```python
from build123d import *

# Parameters (mm, degrees)
SKETCH1_R           = 40
BOSS_EXTRUDE1_DEPTH = 5
CUT_EXTRUDE3_START  = -10
CUT_EXTRUDE3_DEPTH  = 10
FILLET1_R           = 30
FILLET2_R           = 25
SKETCH14_W          = 7
SKETCH14_H          = 5.05
CUT_EXTRUDE4_DEPTH  = 10
SKETCH18_W          = 10
SKETCH18_H          = 7
CUT_EXTRUDE6_DEPTH  = 10
SKETCH20_R          = 8.5
CUT_EXTRUDE8_DEPTH  = 1


with BuildPart() as part:
    # Sketch1 → Boss-Extrude1 (new body)
    with BuildSketch(Plane.XY):
        Circle(SKETCH1_R)
    extrude(amount=BOSS_EXTRUDE1_DEPTH)

    # Sketch10 → Cut-Extrude3 (cut)
    with BuildSketch(Plane.XY.offset(5).offset(CUT_EXTRUDE3_START)):
        with BuildLine():
            Line((-30, 26.457513111), (-30, -26.457513111))
            ThreePointArc((-30, -26.457513111), (-40, 0), (-30, 26.457513111))
        make_face()
        with BuildLine():
            Line((30, 26.457513111), (30, -26.457513111))
            ThreePointArc((30, -26.457513111), (40, 0), (30, 26.457513111))
        make_face()
    extrude(amount=CUT_EXTRUDE3_DEPTH, mode=Mode.SUBTRACT)

    # Fillet1
    fillet1_edges = [part.edges().sort_by_distance(p)[0] for p in [
        (-30, 26.457513111, 2.5),
        (30, 26.457513111, 2.5),
    ]]
    fillet(fillet1_edges, radius=FILLET1_R - 0.0001)  # a hair under: the kernel refuses the full size

    # Fillet2
    fillet2_edges = [part.edges().sort_by_distance(p)[0] for p in [
        (-30, -26.457513111, 2.5),
        (30, -26.457513111, 2.5),
    ]]
    fillet(fillet2_edges, radius=FILLET2_R)

    # Sketch14 → Cut-Extrude4 (cut)
    with BuildSketch(Plane.XY.offset(5)):
        with Locations((0, 1.975)):
            Rectangle(SKETCH14_W, SKETCH14_H)
        with Locations((0, -18.075)):
            Rectangle(SKETCH14_W, SKETCH14_H)
    extrude(amount=-CUT_EXTRUDE4_DEPTH, mode=Mode.SUBTRACT)

    # Sketch18 → Cut-Extrude6 (cut)
    with BuildSketch(Plane(origin=(0, 0, 0), x_dir=(-1, 0, 0), z_dir=(0, 0, -1))):
        with Locations((-18, -7)):
            Rectangle(SKETCH18_W, SKETCH18_H)
    extrude(amount=-CUT_EXTRUDE6_DEPTH, mode=Mode.SUBTRACT)

    # Sketch20 → Cut-Extrude8 (cut)
    with BuildSketch(Plane(origin=(0, 0, 0), x_dir=(-1, 0, 0), z_dir=(0, 0, -1))):
        with Locations((-17.5, 20)):
            Circle(SKETCH20_R)
        with Locations((17.5, 20)):
            Circle(SKETCH20_R)
        with Locations((17.5, -20)):
            Circle(SKETCH20_R)
        with Locations((-17.5, -20)):
            Circle(SKETCH20_R)
    extrude(amount=-CUT_EXTRUDE8_DEPTH, mode=Mode.SUBTRACT)


solid = part.part
```
Could you check a few things on this model? Use its own coordinates, in mm. A direction names the side the tool comes from. Coordinates: 2 decimals unless noted, no trailing zeros. Order: outer loops, then holes, each group sorted by start corner. A loop starts at its lowest first (then second) coordinate and runs counter-clockwise, first axis right, second up. Notation, with made-up numbers: M -12,47 L -8,47 A6 cw -8,54 Z; hole C -1,-27 d1. An arc over 180 degrees is marked long. Use one line per item in the form item = value. Start each with the question number.
1. Suppose I cut it at D-D on x = -17.5. Write out the boundary of the cut face in (y, z), then the cut area to 3 significant figures.
2. For pin 1 (3 mm diameter, centred on y = 17.5, z = 3.5, fed in from +X); pin 2 (5 mm diameter, centred on x = -19, y = 24, fed in from -Z); pin 3 (2.5 mm diameter, centred on y = -17.5, z = 2, fed in from +X), each with a flat end and sliding along its axis, tell me the tip position at first contact or that it passes through.
3. Suppose I cut it at C-C on y = 20. Write out the boundary of the cut face in (x, z).
4. Please list where these lines run through material, in increasing order: line 1 (Y direction, x = -17.5, z = 0.8); line 2 (Y direction, x = 2, z = 3.1); line 3 (X direction, y = 1, z = 2.25).
5. Suppose I cut it at B-B on x = 17.5. Write out the boundary of the cut face in (y, z), then the cut area to 3 significant figures.
6. On a 3-axis mill with a long thin cutter (end or side, diameter ignored), from which of +Z, -Z, +X, -X, +Y, -Y can I reach the whole of each face in a straight line? I mean faces 4 (the cylindrical face through (-10.755, 14.828, 0.493)), 5 (the flat face through (18, -3.5, 2)), 6 (the cylindrical face through (20.979, 31.445, 2.535)). Say none if no direction works.
7. Suppose I cut it at A-A on z = 2.3. Count the separate pieces of the cut face and the enclosed holes in it, then the cut area to 3 significant figures.
8. We'd pull the mould along Y, two halves only. Please class faces 1 (the flat face through (6, 1, 0)), 2 (the flat face through (0, 4.5, 3)), 3 (the cylindrical face through (-20.979, 31.445, 2.535)): +Y half, -Y half, draft (parallel to the pull), parting line (faces both ways), or undercut.
Geometry says:
q1.outline = M -35.79,0 L -28.5,0 L -28.5,1 L -11.5,1 L -11.5,0 L 11.5,0 L 11.5,1 L 28.5,1 L 28.5,0 L 34.37,0 L 34.37,5 L -35.79,5 Z
q1.area = 317 mm^2
q2.pin_1 = 29.39
q2.pin_2 = 1
q2.pin_3 = 29.91
q3.outline = M -28.28,0 L -26,0 L -26,1 L -9,1 L -9,0 L 9,0 L 9,1 L 26,1 L 26,0 L 28.28,0 L 28.28,5 L -28.28,5 Z
q4.line_1 = -35.79 to -28.5, -11.5 to 11.5, 28.5 to 34.37
q4.line_2 = -39.95 to -20.6, -15.55 to -0.55, 4.5 to 39.93
q4.line_3 = -30 to -3.5, 3.5 to 30
q5.outline = M -35.79,0 L -28.5,0 L -28.5,1 L -11.5,1 L -11.5,0 L -10.5,0 L -10.5,5 L -35.79,5 Z; M -3.5,0 L 11.5,0 L 11.5,1 L 28.5,1 L 28.5,0 L 34.37,0 L 34.37,5 L -3.5,5 Z
q5.area = 282 mm^2
q6.face_4 = -Z
q6.face_5 = +Z, -Z
q6.face_6 = +Z, -Z, +X, +Y
q7.separate_pieces = 1
q7.enclosed_holes = 3
q7.area = 3,960 mm^2
q8.face_1 = draft
q8.face_2 = undercut
q8.face_3 = +Y half
